CAD build for the part. Positions are in the model's coordinates, mm. A direction names the side the tool comes from. Round coordinates to 2 decimals unless told otherwise and drop trailing zeros. Order: outer loops, then holes, each group sorted by start corner. A loop starts at its lowest first (then second) coordinate and runs counter-clockwise, first axis right, second up. Notation, with made-up numbers: (76.5, -18) - (133.5, -18) arc R23 ccw to (133.5, -8) - close; hole circle Ø6 at (58.25, 73). An arc over 180 degrees is marked (long way). Use one line per item in the form item = value. Start each with the question number.
from build123d import *

# Parameters (mm, degrees)
F0_W      = 50
F0_H      = 60
F1_DEPTH  = 1.5
F2_W      = 20
F2_H      = 2
F3_DEPTH  = 9
F4_W      = 6
F4_H      = 5.5
F5_DEPTH  = 32
F6_W      = 35
F6_H      = 35
F7_DEPTH  = 4.5
F8_R      = 3
F9_DEPTH  = 5
F10_DEPTH = 5
F11_DEPTH = 5
F12_DEPTH = 5
F13_R     = 1
F14_R     = 0.5


with BuildPart() as f1:
    # F0 (on Top) → F1 (new body)
    with BuildSketch(Plane.XY):
        Rectangle(F0_W, F0_H)
    extrude(amount=F1_DEPTH)

    # F2 (on Top) → F3 (join)
    with BuildSketch(Plane.XY):
        with Locations((10, 31)):
            Rectangle(F2_W, F2_H)
        with Locations((-10, 31)):
            Rectangle(F2_W, F2_H)
        with Locations((-10, -31)):
            Rectangle(F2_W, F2_H)
        with Locations((10, -31)):
            Rectangle(F2_W, F2_H)
    extrude(amount=F3_DEPTH)

    # F4 (on Front) → F5 (cut, symmetric)
    with BuildSketch(Plane.XZ):
        with Locations((-14.75, 4.25)):
            Rectangle(F4_W, F4_H)
        with Locations((14.75, 4.25)):
            Rectangle(F4_W, F4_H)
    extrude(amount=F5_DEPTH, both=True, mode=Mode.SUBTRACT)

    # F6 (on Top) → F7 (join)
    with BuildSketch(Plane.XY):
        Rectangle(F6_W, F6_H)
    extrude(amount=F7_DEPTH)

    # F8
    f8_edges = [f1.edges().sort_by_distance(p)[0] for p in [
        (17.5, -17.5, 3),
        (-17.5, -17.5, 3),
        (-17.5, 17.5, 3),
        (17.5, 17.5, 3),
    ]]
    fillet(f8_edges, radius=F8_R)

    # F9 (add): a face of the model
    f9_faces = [f1.faces().sort_by_distance(p)[0] for p in [
        (20, -31, 4.5),
    ]]
    extrude(f9_faces, amount=F9_DEPTH)

    # F10 (add): a face of the model
    f10_faces = [f1.faces().sort_by_distance(p)[0] for p in [
        (-20, 31, 4.5),
    ]]
    extrude(f10_faces, amount=F10_DEPTH)

    # F11 (add): a face of the model
    f11_faces = [f1.faces().sort_by_distance(p)[0] for p in [
        (-20, -31, 4.5),
    ]]
    extrude(f11_faces, amount=F11_DEPTH)

    # F12 (add): a face of the model
    f12_faces = [f1.faces().sort_by_distance(p)[0] for p in [
        (20, 31, 4.5),
    ]]
    extrude(f12_faces, amount=F12_DEPTH)

    # F13
    f13_edges = [f1.edges().sort_by_distance(p)[0] for p in [
        (25, 31, 9),
        (-25, -31, 9),
        (-25, 31, 9),
        (25, -31, 9),
    ]]
    fillet(f13_edges, radius=F13_R)

    # F14
    f14_edges = [f1.edges().sort_by_distance(p)[0] for p in [
        (-21.375, 30, 1.5),
        (21.375, 30, 1.5),
        (0, 30, 1.5),
        (-21.375, -30, 1.5),
        (0, -30, 1.5),
        (21.375, -30, 1.5),
        (0, 30, 9),
        (-24.707107, 30, 8.707107),
        (24.707107, 30, 8.707107),
        (-25, 30, 4.75),
        (-25, 0, 1.5),
        (-25, -30, 4.75),
        (25, -30, 4.75),
        (25, 0, 1.5),
        (25, 30, 4.75),
        (-24.707107, -30, 8.707107),
        (0, -30, 9),
        (24.707107, -30, 8.707107),
    ]]
    fillet(f14_edges, radius=F14_R)


solid = f1.part
(1) Slice it at D-D (x = 16). Give the cut face in (y, z), and give its area (3 significant figures).
(2) Slice it at A-A (z = 5.75). Give the cut face in (x, y), and give its area (3 significant figures).
(3) Flat gauge pins, fed straight in: P1, Ø1.5, axis at x = 5, y = -18.5, coming from the +Z side; P2, Ø0.9, axis at y = 0.5, z = 2.5, coming from the +X side; P3, Ø3.5, axis at y = 2, z = 3.5, coming from the -X side. Where does each tip first touch, or does it go through?
(4) Which spindle directions (+Z, -Z, +X, -X, +Y, -Y) get a long thin tool onto all of the face, cutting with end or side? Do faces 4 (the flat face through (0, -17.5, 3)), 5 (the flat face through (11.75, -31, 4)), 6 (the flat face through (-17.75, -31, 4)), 7 (the flat face through (-17.5, 0, 3)). Say none if no direction does.
(5) Slice it at B-B (y = 3.5). Give the cut face in (x, z).
(6) Mould opens along Z. For faces 1 (the flat face through (0, 0, 0)), 2 (the flat face through (0, -31, 9)), 3 (the flat face through (11.75, 31, 4)) say: pulls with the +Z half, pulls with the -Z half, needs draft (parallel to the pull), parting line crosses it, or undercut.
(7) Wall check: line 1 (Y direction, x = -2.5, z = 4.25); line 2 (Y direction, x = -6.5, z = 8); line 3 (Z direction, x = -15, y = -9.5). Give the ranges that are in metal, low to high. Write a range as [from, to].
(8) Slice it at C-C (x = 4.5). Give the cut face in (y, z).
Results list:
q1.outline = (-32, 0) - (32, 0) - (32, 1.5) - (17.1, 1.5) - (17.1, 4.5) - (-17.1, 4.5) - (-17.1, 1.5) - (-32, 1.5) - close; (-32, 7) - (-30, 7) - (-30, 8.5) arc R0.5 ccw to (-30.5, 9) - (-32, 9) - close; (30, 7) - (32, 7) - (32, 9) - (30.5, 9) arc R0.5 ccw to (30, 8.5) - close
q1.area = 206 mm²
q2.outline = (-25, -32) - (-17.75, -32) - (-17.75, -30) - (-24.5, -30) arc R0.5 ccw to (-25, -30.5) - close; (-25, 30.5) arc R0.5 ccw to (-24.5, 30) - (-17.75, 30) - (-17.75, 32) - (-25, 32) - close; (-11.75, -32) - (11.75, -32) - (11.75, -30) - (-11.75, -30) - close; (-11.75, 30) - (11.75, 30) - (11.75, 32) - (-11.75, 32) - close; (17.75, -32) - (25, -32) - (25, -30.5) arc R0.5 ccw to (24.5, -30) - (17.75, -30) - close; (17.75, 30) - (24.5, 30) arc R0.5 ccw to (25, 30.5) - (25, 32) - (17.75, 32) - close
q2.area = 152 mm²
q3.P1 = 1.5
q3.P2 = 17.5
q3.P3 = -17.5
q4.face_4 = +Z, +X, -X
q4.face_5 = -Y
q4.face_6 = +Y, -Y
q4.face_7 = +Z, -X, +Y, -Y
q5.outline = (-25, 0) - (25, 0) - (25, 1) arc R0.5 ccw to (24.5, 1.5) - (17.5, 1.5) - (17.5, 4.5) - (-17.5, 4.5) - (-17.5, 1.5) - (-24.5, 1.5) arc R0.5 ccw to (-25, 1) - close
q6.face_1 = pulls with the -Z half
q6.face_2 = pulls with the +Z half
q6.face_3 = undercut
q7.line_1 = [-32, -30], [-17.5, 17.5], [30, 32]
q7.line_2 = [-32, -30], [30, 32]
q7.line_3 = [0, 4.5]
q8.outline = (-32, 0) - (32, 0) - (32, 9) - (30.5, 9) arc R0.5 ccw to (30, 8.5) - (30, 2) arc R0.5 cw to (29.5, 1.5) - (17.5, 1.5) - (17.5, 4.5) - (-17.5, 4.5) - (-17.5, 1.5) - (-29.5, 1.5) arc R0.5 cw to (-30, 2) - (-30, 8.5) arc R0.5 ccw to (-30.5, 9) - (-32, 9) - close
